Autodesk Inventor part; units mm, degrees
ref_plane "YZ Plane" through (0, 0, 0) normal (1, 0, 0) x (0, 1, 0)
ref_plane "XZ Plane" through (0, 0, 0) normal (0, 1, 0) x (-1, 0, 0)
ref_plane "XY Plane" through (0, 0, 0) normal (0, 0, 1) x (1, 0, 0)
sketch "Boceto1" plane through (0, 0, 0) normal (0, 0, 1) x (1, 0, 0)
  line L0 (0, 200) -> (300, 200)
  line L1 (25, 0) -> (25, 3)
  line L2 (25, 3) -> (125, 3)
  line L3 (125, 3) -> (125, 0)
  line L4 (175, 0) -> (175, 3)
  line L5 (175, 3) -> (275, 3)
  line L6 (275, 3) -> (275, 0)
  line L7 (25, 0) -> (0, 0)
  line L8 (300, 0) -> (275, 0)
  line L9 (175, 0) -> (125, 0)
  line L10 (0, 150) -> (-3, 150)
  line L11 (-3, 150) -> (-3, 50)
  line L12 (-3, 50) -> (0, 50)
  line L13 (0, 0) -> (0, 50)
  line L14 (0, 150) -> (0, 200)
  line L15 (300, 150) -> (303, 150)
  line L16 (303, 150) -> (303, 50)
  line L17 (303, 50) -> (300, 50)
  line L18 (300, 200) -> (300, 150)
  line L19 (300, 50) -> (300, 0)
  dimension "d4" = 100
  dimension "d6" = 100
  dimension "d10" = 50
  dimension "d13" = 3
  dimension "d14" = 200
  dimension "d15" = 3
  dimension "d16" = 100
  dimension "d17" = 50
  dimension "d21" = 300
extrude "Extrusión1" add sketch "Boceto1" along normal blind 3
sketch "Boceto2" plane through (0, 0, 3) normal (0, 0, 1) x (1, 0, 0)
  line L0 (68.5, 53) -> (218.5, 53)
  line L1 (218.5, 53) -> (218.5, 13)
  line L2 (218.5, 13) -> (68.5, 13)
  line L3 (68.5, 13) -> (68.5, 53)
  line L4 (0, 50) -> (0, 0)
  line L5 (25, 3) -> (125, 3)
  dimension "d22" = 40
  dimension "d23" = 150
  dimension "d26" = 68.5
  dimension "d27" = 10
extrude "Extrusión2" cut sketch "Boceto2" against normal blind 3
properties part number "Base lateral"
The listing builds one solid part. Answer for the finished solid, in the listing's coordinates (mm). Coordinates: 2 decimals unless noted, no trailing zeros. Loops run counter-clockwise (first coordinate to the right, second up) from the corner with the lowest first, then second, coordinate; pieces in that order, holes last. Notation, with made-up numbers: (85, -28) -> (143, -28) arc R19 ccw to (143, -6) -> close; hole circle Ø1 at (81.25, 16.25). An arc over 180 degrees is marked (long way). Write item = value, one per line. Start each with the question number.
1) A cutting plane is placed at C-C (z = 1.6). Give the vertices of the cut face in (x, y).
2) Given pin 1 Ø1.5 at (y, z) = (1, 1) entering from -X; pin 2 Ø0.9 at (y, z) = (24, 2) entering from +X; pin 3 Ø1 at (x, z) = (45, 2.5) entering from -Y, each flat-ended and moving along its own axis, determine where each tip first touches the part or whether it passes through.
3) Straight lines are drawn through the part: line 1 (Y direction, x = 109, z = 2.55); line 2 (Y direction, x = 174.5, z = 1.4); line 3 (X direction, y = 44.5, z = 0.75). For each, find the intervals that lie inside material, in ascending order. Write a range as from..to.
4) A cutting plane is placed at B-B (x = 130). Give the vertices of the cut face in (y, z).
5) A cutting plane is placed at A-A (y = 38.5). Give the vertices of the cut face in (x, z), then the cut area to 3 significant figures.
Responses:
q1.outline = (-3, 50) -> (0, 50) -> (0, 0) -> (25, 0) -> (25, 3) -> (125, 3) -> (125, 0) -> (175, 0) -> (175, 3) -> (275, 3) -> (275, 0) -> (300, 0) -> (300, 50) -> (303, 50) -> (303, 150) -> (300, 150) -> (300, 200) -> (0, 200) -> (0, 150) -> (-3, 150) -> close; hole (68.5, 13) -> (218.5, 13) -> (218.5, 53) -> (68.5, 53) -> close
q2.pin_1 = 0
q2.pin_2 = 300
q2.pin_3 = 3
q3.line_1 = 3..13, 53..200
q3.line_2 = 0..13, 53..200
q3.line_3 = 0..68.5, 218.5..300
q4.outline = (0, 0) -> (13, 0) -> (13, 3) -> (0, 3) -> close; (53, 0) -> (200, 0) -> (200, 3) -> (53, 3) -> close
q5.outline = (0, 0) -> (68.5, 0) -> (68.5, 3) -> (0, 3) -> close; (218.5, 0) -> (300, 0) -> (300, 3) -> (218.5, 3) -> close
q5.area = 450 mm²
